from build123d import *

# Parameters (mm, degrees)
F0_R     = 13.5
F1_DEPTH = 7
F2_W     = 9.5
F2_H     = 9.5
F3_DEPTH = 4.5
F4_R     = 1.5
F5_DEPTH = 25.4
F8_DEPTH = 0.1


with BuildPart() as f1:
    # F0 (on Top) → F1 (new body)
    with BuildSketch(Plane.XY):
        Circle(F0_R)
    extrude(amount=F1_DEPTH)

    # F2 (on Top) → F3 (cut)
    with BuildSketch(Plane.XY):
        Rectangle(F2_W, F2_H)
    extrude(amount=F3_DEPTH, mode=Mode.SUBTRACT)

    # F4 (on Top) → F5 (cut)
    with BuildSketch(Plane.XY):
        with Locations((13.5, 0)):
            Circle(F4_R)
        with Locations((-13.5, 0)):
            Circle(F4_R)
        with Locations((0, -13.5)):
            Circle(F4_R)
        with Locations((0, 13.5)):
            Circle(F4_R)
        with BuildLine():
            ThreePointArc((-8.045941546, 9.545941546), (-8.9719163975, 10.9317608448), (-10.6066017178, 10.6066017178))
            Line((-10.6066017178, 10.6066017178), (-8.4852813742, 8.4852813742))
            ThreePointArc((-8.4852813742, 8.4852813742), (-8.1601222473, 8.9719163975), (-8.045941546, 9.545941546))
        make_face()
        with BuildLine():
            ThreePointArc((10.6066017178, 10.6066017178), (8.4852813742, 10.6066017178), (8.4852813742, 8.4852813742))
            Line((8.4852813742, 8.4852813742), (10.6066017178, 10.6066017178))
        make_face()
        with BuildLine():
            Line((10.6066017178, 10.6066017178), (8.4852813742, 8.4852813742))
            ThreePointArc((8.4852813742, 8.4852813742), (10.1199666946, 8.1601222473), (11.045941546, 9.545941546))
            ThreePointArc((11.045941546, 9.545941546), (10.9317608448, 10.1199666946), (10.6066017178, 10.6066017178))
        make_face()
        with BuildLine():
            ThreePointArc((11.045941546, -9.545941546), (10.1199666946, -8.1601222473), (8.4852813742, -8.4852813742))
            Line((8.4852813742, -8.4852813742), (10.6066017178, -10.6066017178))
            ThreePointArc((10.6066017178, -10.6066017178), (10.9317608448, -10.1199666946), (11.045941546, -9.545941546))
        make_face()
        with BuildLine():
            Line((10.6066017178, -10.6066017178), (8.4852813742, -8.4852813742))
            ThreePointArc((8.4852813742, -8.4852813742), (8.4852813742, -10.6066017178), (10.6066017178, -10.6066017178))
        make_face()
        with BuildLine():
            ThreePointArc((-8.045941546, -9.545941546), (-8.1601222473, -8.9719163975), (-8.4852813742, -8.4852813742))
            Line((-8.4852813742, -8.4852813742), (-10.6066017178, -10.6066017178))
            ThreePointArc((-10.6066017178, -10.6066017178), (-8.9719163975, -10.9317608448), (-8.045941546, -9.545941546))
        make_face()
        with BuildLine():
            Line((-10.6066017178, -10.6066017178), (-8.4852813742, -8.4852813742))
            ThreePointArc((-8.4852813742, -8.4852813742), (-10.6066017178, -8.4852813742), (-10.6066017178, -10.6066017178))
        make_face()
        with BuildLine():
            Line((-8.4852813742, 8.4852813742), (-10.6066017178, 10.6066017178))
            ThreePointArc((-10.6066017178, 10.6066017178), (-10.6066017178, 8.4852813742), (-8.4852813742, 8.4852813742))
        make_face()
    extrude(amount=F5_DEPTH, mode=Mode.SUBTRACT)

    # F7 (on offset) → F8 (cut)
    with BuildSketch(Plane.XY.offset(7)):
        with BuildLine():
            ThreePointArc((-0.5, 8.5), (0, 8), (0.5, 8.5))
            Line((0.5, 8.5), (-0.5, 8.5))
        make_face()
        with BuildLine():
            Line((-0.5, 8.5), (0.5, 8.5))
            ThreePointArc((0.5, 8.5), (0, 9), (-0.5, 8.5))
        make_face()
        with BuildLine():
            Line((0.5, 3.5), (0.5, 8.5))
            ThreePointArc((0.5, 8.5), (0, 8), (-0.5, 8.5))
            Line((-0.5, 8.5), (-0.5, 3.5))
            ThreePointArc((-0.5, 3.5), (0, 4), (0.5, 3.5))
        make_face()
        with BuildLine():
            ThreePointArc((-0.5, 3.5), (0, 3), (0.5, 3.5))
            Line((0.5, 3.5), (-0.5, 3.5))
        make_face()
        with BuildLine():
            Line((-0.5, 3.5), (0.5, 3.5))
            ThreePointArc((0.5, 3.5), (0, 4), (-0.5, 3.5))
        make_face()
    extrude(amount=-F8_DEPTH, mode=Mode.SUBTRACT)


solid = f1.part
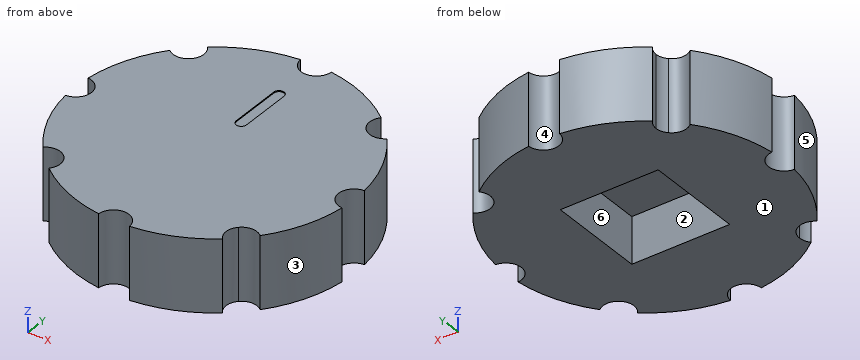
Work out the finished part from the listing and answer in its coordinate system (mm). Face numbers are marked on the shaded views. A direction names the side the tool comes from. Coordinates: 2 decimals unless noted, no trailing zeros. Loops run counter-clockwise (first coordinate to the right, second up) from the corner with the lowest first, then second, coordinate; pieces in that order, holes last. Notation, with made-up numbers: M 31.5,-37 L 66.5,-37 A11 cw 66.5,-25 Z; hole C 25,-0.75 d4. An arc over 180 degrees is marked long. Answer in a Markdown table with one row per item. Add a question column.
1. Consider L1, parallel to Y at x = -8.25, z = 1.25; L2, parallel to Z at x = 0, y = 6. Determine where each line is inside the solid, lowest interval first.
2. Find section B-B, the plane z = 3.5. Write down the section's boundary in (x, y).
3. Find section C-C, the plane x = 0. Write down the section's boundary in (y, z).
4. A tool of negligible diameter and unlimited length cuts with its end or side. For the marked faces 5 and 6, from which of +Z, -Z, +X, -X, +Y, -Y can it reach the whole face along a straight path? Write none if from no direction.
5. Flat-ended cylindrical pins translate along their axes: P1, Ø2, axis at x = 7, z = 5.5, coming from the -Y side; P2, Ø3, axis at y = -8.5, z = 5.5, coming from the -X side; P3, Ø0.8, axis at x = 0, y = 6.5, coming from the +Z side. Find the tip coordinate at first contact, or state that the pin passes through.
6. Find section A-A, the plane y = 0. Write down the section's boundary in (x, z).
7. The mould has two halves that part along X. Classify the marked faces 1, 2, 3 and 4: pulls with the +X half, pulls with the -X half, needs draft (parallel to the pull), parting line crosses it, or undercut.
8. Find section D-D, the plane y = 5.75. Write down the section's boundary in (x, z), then the cut area to 3 significant figures.
Reported:
| question | item | result |
|---|---|---|
| 1 | L1 | y = -10.69 to -10.3, -8.79 to 8.79, 10.3 to 10.69 |
| 1 | L2 | z = 0 to 6.9 |
| 2 | outline | M -13.42,-1.5 A13.5 ccw -10.55,-8.43 A1.5 cw -8.43,-10.55 A13.5 ccw -1.5,-13.42 A1.5 cw 1.5,-13.42 A13.5 ccw 8.43,-10.55 A1.5 cw 10.55,-8.43 A13.5 ccw 13.42,-1.5 A1.5 cw 13.42,1.5 A13.5 ccw 10.55,8.43 A1.5 cw 8.43,10.55 A13.5 ccw 1.5,13.42 A1.5 cw -1.5,13.42 A13.5 ccw -8.43,10.55 A1.5 cw -10.55,8.43 A13.5 ccw -13.42,1.5 A1.5 cw Z; hole M -4.75,-4.75 L 4.75,-4.75 L 4.75,4.75 L -4.75,4.75 Z |
| 3 | outline | M -12,0 L -4.75,0 L -4.75,4.5 L 4.75,4.5 L 4.75,0 L 12,0 L 12,7 L 9,7 L 9,6.9 L 3,6.9 L 3,7 L -12,7 Z |
| 4 | face 5 | +Z, -Z, -X, -Y |
| 4 | face 6 | -Z |
| 5 | P1 | stops at y = -12.09 |
| 5 | P2 | stops at x = -11.54 |
| 5 | P3 | stops at z = 6.9 |
| 6 | outline | M -12,0 L -4.75,0 L -4.75,4.5 L 4.75,4.5 L 4.75,0 L 12,0 L 12,7 L -12,7 Z |
| 7 | face 1 | needs draft |
| 7 | face 2 | undercut |
| 7 | face 3 | pulls with the +X half |
| 7 | face 4 | undercut |
| 8 | outline | M -12.21,0 L 12.21,0 L 12.21,7 L 0.5,7 L 0.5,6.9 L -0.5,6.9 L -0.5,7 L -12.21,7 Z |
| 8 | area | 171 mm^2 |
